from build123d import *

# Parameters (mm, degrees)
SKETCH1_R           = 1
BOSS_EXTRUDE1_DEPTH = 11.975
SKETCH2_W           = 20
SKETCH2_H           = 23.8
SKETCH2_R           = 1.575
SKETCH2_R_2         = 2.25
BOSS_EXTRUDE2_DEPTH = 2
SKETCH3_W           = 23.95
SKETCH3_H           = 20
BOSS_EXTRUDE3_DEPTH = 2
SKETCH4_W           = 20
SKETCH4_H           = 19.8
CUT_EXTRUDE1_DEPTH  = 19


with BuildPart() as part:
    # Sketch1 → Boss-Extrude1 (new, symmetric)
    with BuildSketch(Plane(origin=(0, 0, 0), x_dir=(0, 0, -1), z_dir=(1, 0, 0))):
        with BuildLine():
            Line((21.768222654, 1.933048137), (-79.231777346, 1.933048137))
            ThreePointArc((-79.231777346, 1.933048137), (-80.645990908, 1.347261699), (-81.231777346, -0.066951863))
            Line((-81.231777346, -0.066951863), (-81.231777346, -1.066951863))
            ThreePointArc((-81.231777346, -1.066951863), (-78.231777346, -4.066951863), (-75.231777346, -1.066951863))
            Line((-75.231777346, -1.066951863), (21.768222654, -1.066951863))
            Line((21.768222654, -1.066951863), (21.768222654, 1.933048137))
        make_face()
        with Locations((-78.231777346, -1.066951863)):
            Circle(SKETCH1_R, mode=Mode.SUBTRACT)
    extrude(amount=BOSS_EXTRUDE1_DEPTH, both=True)

    # Sketch2 → Boss-Extrude2 (add)
    with BuildSketch(Plane(origin=(11.975, 0, 0), x_dir=(0, 0, -1), z_dir=(1, 0, 0))):
        with Locations((-6.431536694, 13.833048137)):
            Rectangle(SKETCH2_W, SKETCH2_H)
        with Locations((-11.981536694, 4.308048137)):
            Circle(SKETCH2_R, mode=Mode.SUBTRACT)
        with Locations((-11.981536694, 21.558048137)):
            Circle(SKETCH2_R, mode=Mode.SUBTRACT)
        with Locations((-1.231536694, 13.033048137)):
            Circle(SKETCH2_R_2, mode=Mode.SUBTRACT)
    boss_extrude2 = extrude(amount=-BOSS_EXTRUDE2_DEPTH)

    # Mirror1: Boss-Extrude2 across plane
    add(boss_extrude2.mirror(Plane(origin=(0, 0, 0), x_dir=(0, 0, 1), z_dir=(1, 0, 0))))

    # Sketch3 → Boss-Extrude3 (add)
    with BuildSketch(Plane(origin=(0, 25.733048137, 0), x_dir=(1, 0, 0), z_dir=(0, 1, 0))):
        with Locations((0, -6.431536694)):
            Rectangle(SKETCH3_W, SKETCH3_H)
    extrude(amount=BOSS_EXTRUDE3_DEPTH)

    # Sketch4 → Cut-Extrude1 (cut)
    with BuildSketch(Plane(origin=(11.975, 0, 0), x_dir=(0, 0, -1), z_dir=(1, 0, 0))):
        with Locations((-6.431536694, 17.833048137)):
            Rectangle(SKETCH4_W, SKETCH4_H)
    extrude(amount=-CUT_EXTRUDE1_DEPTH, mode=Mode.SUBTRACT)


solid = part.part
Verification items for the finished model (mm, model axes). A direction names the side the tool comes from. Round coordinates to 2 decimals unless told otherwise and drop trailing zeros. Loops run counter-clockwise (first coordinate to the right, second up) from the corner with the lowest first, then second, coordinate; pieces in that order, holes last. Notation, with made-up numbers: M 17,34 L 76,34 A12 cw 76,47 Z; hole C 63,20 d9. An arc over 180 degrees is marked long. Write each question's results on one line, items separated by ' | '.
1) Scan lines: L1, parallel to Y at x = 8.25, z = 73.5; L2, parallel to X at y = 17, z = 4 (3 decimals); L3, parallel to Z at x = 10.25, y = 7.5. Record each from-to range of solid material in increasing order. Write a range as from..to.
Checks:
L1: y = -1.07..1.93 | L2: x = -11.975..-9.975 | L3: z = -3.57..16.43
2) Section check A-A on x = 8.5. Record the boundary of the cut face in (y, z), then the cut area to 3 significant figures.
Checks:
outline: M -1.07,-21.77 L 1.93,-21.77 L 1.93,79.23 A2 ccw -0.07,81.23 L -1.07,81.23 A3 ccw -1.07,75.23 Z; hole C -1.07,78.23 d2 | area: 319 mm2
3) Access from +Z, -Z, +X, -X, +Y, -Y to the whole of each face (thin tool, end or side, straight path). Record for faces 1 (the flat face through (11, 5, -3.568)), 2 (the flat face through (-11, 15, 16.432)), 3 (the flat face through (9.975, 5, 7)), 4 (the flat face through (11, 7.933, 7)), 5 (the cylindrical face through (-10.99, 20.02, 12.32)).
Checks:
face 1: -Z, +X, -X, +Y | face 2: +Z, +X, -X, +Y | face 3: +Z, -Z, +Y | face 4: +Z, -Z, +X, +Y | face 5: +X, -X
4) Mould release check, pull along Z, two halves, no side actions. Record for faces 6 (the flat face through (-10, 27.733, 6)), 7 (the cylindrical face through (-10.99, 11.04, 0.19)), 8 (the flat face through (-11, 15, -3.568)): released by +Z, released by -Z, zero draft, split by the parting line, or undercut.
Checks:
face 6: zero draft | face 7: undercut | face 8: released by -Z
5) Gauge pin test, flat ends, axial feed: P1, Ø8, axis at x = 1.5, z = -10, coming from the +Y side; P2, Ø5, axis at y = 13.03, z = 1.23, coming from the +X side (3 decimals); P3, Ø8, axis at y = 22.5, z = -3, coming from the +X side (3 decimals); P4, Ø3.5, axis at y = 4.31, z = 11.98, coming from the -X side (3 decimals). Record the tip position at first contact, or that the pin passes through.
Checks:
P1: stops at y = 1.93 | P2: stops at x = -9.975 | P3: stops at x = -7.025 | P4: stops at x = -11.975
6) Section check B-B on z = 2.5. Record the boundary of the cut face in (x, y) (3 decimals).
Checks:
outline: M -11.975,-1.067 L 11.975,-1.067 L 11.975,7.933 L 9.975,7.933 L 9.975,1.933 L -9.975,1.933 L -9.975,11.175 L -11.975,11.175 Z; M -11.975,14.891 L -9.975,14.891 L -9.975,25.733 L -7.025,25.733 L -7.025,27.733 L -11.975,27.733 Z
7) Section check C-C on z = 59.5. Record the boundary of the cut face in (x, y) (3 decimals), then the cut area to 4 significant figures.
Checks:
outline: M -11.975,-1.067 L 11.975,-1.067 L 11.975,1.933 L -11.975,1.933 Z | area: 71.85 mm2
